from build123d import *

# Parameters (mm, degrees)
SKETCH1_R               = 15.24
SKETCH1_R_2             = 9.144
BOSS_EXTRUDE1_DEPTH     = 2.667
SKETCH2_R               = 1.4605
CUT_EXTRUDE1_DEPTH      = 23.202854681
BOSS_EXTRUDE2_START     = -2.667
BOSS_EXTRUDE2_OUTLINE_R = 9.144
BOSS_EXTRUDE2_DEPTH     = 5.334


# Read off the part's stored shape, not the designer's step: Boss-Extrude2
with BuildPart() as part:
    # Sketch1 → Boss-Extrude1 (new, symmetric)
    with BuildSketch(Plane.XY):
        Circle(SKETCH1_R)
        Circle(SKETCH1_R_2, mode=Mode.SUBTRACT)
    extrude(amount=BOSS_EXTRUDE1_DEPTH, both=True)

    # Sketch2 → Cut-Extrude1 (cut, through all)
    with BuildSketch(Plane.XY.offset(2.667)):
        with Locations((12.7, 0)):
            Circle(SKETCH2_R)
        with Locations((-12.7, 0)):
            Circle(SKETCH2_R)
    extrude(amount=-CUT_EXTRUDE1_DEPTH, mode=Mode.SUBTRACT)

    # Boss-Extrude2 outline → Boss-Extrude2 (add)
    with BuildSketch(Plane.XY.offset(BOSS_EXTRUDE2_START)):
        Circle(BOSS_EXTRUDE2_OUTLINE_R)
        with BuildLine():
            Line((1.5875, 4.7625), (1.5875, 6.148361062))
            ThreePointArc((1.5875, 6.148361062), (0, -6.35), (-1.5875, 6.148361062))
            Line((-1.5875, 6.148361062), (-1.5875, 4.7625))
            Line((-1.5875, 4.7625), (1.5875, 4.7625))
        make_face(mode=Mode.SUBTRACT)
    extrude(amount=BOSS_EXTRUDE2_DEPTH)


solid = part.part
Model file for the job. Use its own axes, mm. A direction names the side the tool comes from. Coordinates: 2 decimals unless noted, no trailing zeros. Order: outer loops, then holes, each group sorted by start corner. A loop starts at its lowest first (then second) coordinate and runs counter-clockwise, first axis right, second up. Notation, with made-up numbers: (-19, -0.75) -> (17, -0.75) arc R25 cw to (17, 29.25) -> close; hole circle Ø5 at (85, 51). An arc over 180 degrees is marked (long way). Return JSON: item names as keys, results as strings. Group by question number.
Item 1: Saw through at C-C on z = -1.35. Write the cut outline in (x, y), then the cut area to 3 significant figures.
Item 2: Saw through at B-B on x = 0. Write the cut outline in (y, z).
Item 3: Pull direction X, two halves, no side cores. Call faces 1 (the flat face through (7, 0, -2.667)), 2 (the cylindrical face through (0.257, -6.345, -0.037)), 3 (the cylindrical face through (-3.3, -14.88, 0.04)): pulls with the +X half, pulls with the -X half, needs draft (parallel to the pull), parting line crosses it, or undercut.
Item 4: Saw through at D-D on x = 12.7. Write the cut outline in (y, z).
Item 5: Flat gauge pins, fed straight in: P1, Ø0.7, axis at y = 5.5, z = 0, coming from the -X side; P2, Ø1, axis at x = 9, z = -1.5, coming from the -Y side; P3, Ø1.8, axis at x = -12.7, y = 0, coming from the -Z side; P4, Ø2, axis at x = -10, z = 2, coming from the -Y side. Where does each tip first touch, or does it go through?
Item 6: Saw through at A-A on y = 0. Write the cut outline in (x, z).
Item 7: Tool access for faces 4 (the flat face through (7, 0, 2.667)), 5 (the flat face through (1.588, 5, 0)): list every direction of +Z, -Z, +X, -X, +Y, -Y with a clear straight run to the whole face (end or side of a thin tool).
Item 8: Wall check: line 1 along Y through (x, z) = (0, -0.5); line 2 along X through (y, z) = (-1.5, 1.5); line 3 along X through (y, z) = (4.5, 1.4). Give the ranges that are in metal, low to high. Write a range as [from, to].
Values found:
{
 "1": {"outline": "circle Ø30.48 at (0, 0); hole circle Ø2.92 at (-12.7, 0); hole (-1.59, 4.76) -> (-1.59, 6.15) arc R6.35 ccw (long way) to (1.59, 6.15) -> (1.59, 4.76) -> close; hole circle Ø2.92 at (12.7, 0)", "area": "594 mm2"},
 "2": {"outline": "(-15.24, -2.67) -> (-6.35, -2.67) -> (-6.35, 2.67) -> (-15.24, 2.67) -> close; (4.76, -2.67) -> (15.24, -2.67) -> (15.24, 2.67) -> (4.76, 2.67) -> close"},
 "3": {"face 1": "needs draft", "face 2": "undercut", "face 3": "parting line crosses it"},
 "4": {"outline": "(-8.42, -2.67) -> (-1.46, -2.67) -> (-1.46, 2.67) -> (-8.42, 2.67) -> close; (1.46, -2.67) -> (8.42, -2.67) -> (8.42, 2.67) -> (1.46, 2.67) -> close"},
 "5": {"P1": "stops at x = -14.34", "P2": "stops at y = -12.65", "P3": "passes through", "P4": "stops at y = -12.3"},
 "6": {"outline": "(-15.24, -2.67) -> (-14.16, -2.67) -> (-14.16, 2.67) -> (-15.24, 2.67) -> close; (-11.24, -2.67) -> (-6.35, -2.67) -> (-6.35, 2.67) -> (-11.24, 2.67) -> close; (6.35, -2.67) -> (11.24, -2.67) -> (11.24, 2.67) -> (6.35, 2.67) -> close; (14.16, -2.67) -> (15.24, -2.67) -> (15.24, 2.67) -> (14.16, 2.67) -> close"},
 "7": {"face 4": "+Z, +X, -X, +Y, -Y", "face 5": "+Z, -Z"},
 "8": {"line 1": "y = [-15.24, -6.35], [4.76, 15.24]", "line 2": "x = [-15.17, -6.17], [6.17, 15.17]", "line 3": "x = [-14.56, -4.48], [4.48, 14.56]"}
}
